from build123d import *

# Parameters (mm, degrees)
F0_R     = 3.5
F0_W     = 100
F0_H     = 40
F1_DEPTH = 10


with BuildPart() as f1:
    # F0 (on Top) → F1 (new body)
    with BuildSketch(Plane.XY):
        Polygon((300, 175), (300, 375), (-300, 375), (-300, 175), (-270, 175), (-270, 145), (-300, 145), (-300, -215), (-270, -215), (-270, -245), (-300, -245), (-300, -375), (300, -375), (300, -245), (270, -245), (270, -215), (300, -215), (300, 145), (270, 145), (270, 175), align=None)
        with Locations((-285, -360)):
            Circle(F0_R, mode=Mode.SUBTRACT)
        with Locations((-285, -265)):
            Circle(F0_R, mode=Mode.SUBTRACT)
        with Locations((-285, -195)):
            Circle(F0_R, mode=Mode.SUBTRACT)
        with Locations((-250, -230)):
            Circle(F0_R, mode=Mode.SUBTRACT)
        with Locations((0, -360)):
            Circle(F0_R, mode=Mode.SUBTRACT)
        with Locations((285, -360)):
            Circle(F0_R, mode=Mode.SUBTRACT)
        with Locations((285, -265)):
            Circle(F0_R, mode=Mode.SUBTRACT)
        with Locations((250, -230)):
            Circle(F0_R, mode=Mode.SUBTRACT)
        with Locations((285, -195)):
            Circle(F0_R, mode=Mode.SUBTRACT)
        with Locations((-285, 115)):
            Circle(F0_R, mode=Mode.SUBTRACT)
        with Locations((-250, 160)):
            Circle(F0_R, mode=Mode.SUBTRACT)
        with Locations((-285, 195)):
            Circle(F0_R, mode=Mode.SUBTRACT)
        with Locations((-285, 360)):
            Circle(F0_R, mode=Mode.SUBTRACT)
        with Locations((285, 115)):
            Circle(F0_R, mode=Mode.SUBTRACT)
        with Locations((250, 160)):
            Circle(F0_R, mode=Mode.SUBTRACT)
        with Locations((0, 195)):
            Rectangle(F0_W, F0_H, mode=Mode.SUBTRACT)
        with Locations((0, 360)):
            Circle(F0_R, mode=Mode.SUBTRACT)
        with Locations((285, 195)):
            Circle(F0_R, mode=Mode.SUBTRACT)
        with Locations((285, 360)):
            Circle(F0_R, mode=Mode.SUBTRACT)
    extrude(amount=F1_DEPTH)


solid = f1.part
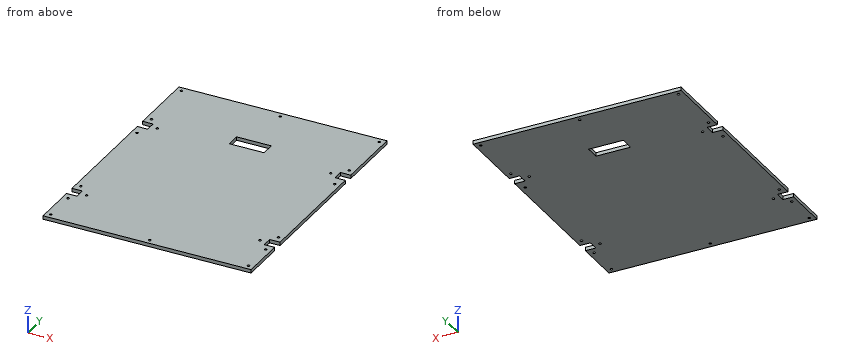
Geometry check sheet. Reference: the model listing, model coordinates, mm. Round coordinates to 2 decimals unless told otherwise and drop trailing zeros. Loops run counter-clockwise (first coordinate to the right, second up) from the corner with the lowest first, then second, coordinate; pieces in that order, holes last.
Item 1: Cross-section at B-B on z = 5.25. Count the separate pieces of the cut face and the enclosed holes in it, then the cut area to 3 significant figures.
Item 2: Gauge pin test, flat ends, axial feed: pin 1 (5.5 mm diameter, centred on x = 285, y = -265, fed in from +Z); pin 2 (5 mm diameter, centred on y = 160.5, z = 3, fed in from -X). Record the tip position at first contact, or that the pin passes through.
Item 3: Cross-section at A-A on x = 33.5. Record the boundary of the cut face in (y, z).
Item 4: Thickness scan on line 1 (Y direction, x = 0, z = 2); line 2 (X direction, y = 160, z = 7.25); line 3 (X direction, y = 360, z = 5.5). Record the ranges inside material, lowest first.
Answer sheet:
1. separate pieces: 1
1. enclosed holes: 19
1. area: 442,000 mm2
2. pin 1: passes through
2. pin 2: stops at x = -270
3. outline: (-375, 0) - (175, 0) - (175, 10) - (-375, 10) - close; (215, 0) - (375, 0) - (375, 10) - (215, 10) - close
4. line 1: y = -375 to -363.5, -356.5 to 175, 215 to 356.5, 363.5 to 375
4. line 2: x = -270 to -253.5, -246.5 to 246.5, 253.5 to 270
4. line 3: x = -300 to -288.5, -281.5 to -3.5, 3.5 to 281.5, 288.5 to 300
